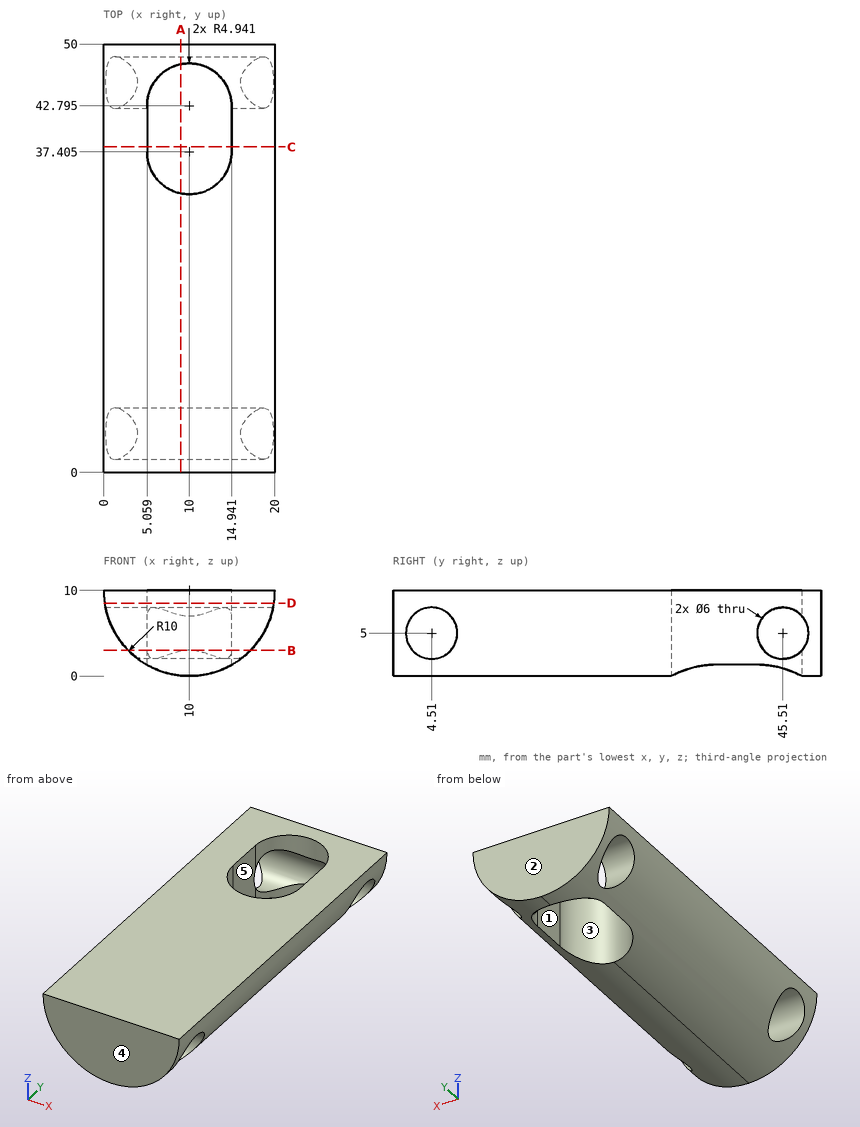
Verification items for this drawing (mm, ordinates from the low corner). A direction names the side the tool comes from. Coordinates: 2 decimals unless noted, no trailing zeros. Write each loop counter-clockwise with the first axis right and the second up, starting at its lowest first coordinate (ties: lowest second). Pieces come first, ordered by that corner, then holes. Notation, with made-up numbers: (1, 83) -> (43, 83) arc R27 cw to (43, 113) -> close; hole circle Ø3 at (4.25, 1.25). An arc over 180 degrees is marked (long way). Use CSV: the item, a comma, the result in double quotes. Start each with the question number.
Item 1: Thickness scan on line 1 (Y direction, x = 8.5, z = 5); line 2 (Y direction, x = 6.5, z = 5); line 3 (Y direction, x = 10.5, z = 1). Record the ranges inside material, lowest first.
Item 2: Depth check by flat-ended pin: pin 1 Ø4 at (y, z) = (24.5, 7) entering from -X; pin 2 Ø2 at (y, z) = (45, 2) entering from +X. Enter the tip coordinate at first touch or a pass-through.
Item 3: Cross-section at D-D, the plane z = 8.5. Record the cut outline in (x, y) (1 decimal).
Item 4: Set-up check for the marked faces 1 and 2: record each of +Z, -Z, +X, -X, +Y, -Y from which the full face is reachable in a straight line by a thin tool's end or side.
Item 5: Cross-section at B-B, the plane z = 3. Record the cut outline in (x, y) (1 decimal), plus the area to 3 significant figures.
Item 6: Cross-section at C-C, the plane y = 38. Record the cut outline in (x, z).
Item 7: Mould release check, pull along X, two halves, no side actions. Record for the marked faces 3, 4 and 5: released by +X, released by -X, zero draft, split by the parting line, or undercut.
Item 8: Cross-section at A-A, the plane x = 9. Record the cut outline in (y, z), plus the area to 3 significant figures.
Answers:
1,line 1,"0 to 1.51, 7.51 to 32.7, 48.51 to 50"
1,line 2,"0 to 1.51, 7.51 to 33.92, 48.51 to 50"
1,line 3,"0 to 32.49, 47.71 to 50"
2,pin 1,"x = 0.05"
2,pin 2,"x = 16.46"
3,outline,"(0.1, 0) -> (19.9, 0) -> (19.9, 50) -> (0.1, 50) -> close; hole (5.1, 37.4) arc R4.9 ccw to (14.9, 37.4) -> (14.9, 42.8) arc R4.9 ccw to (5.1, 42.8) -> close"
4,face 1,"+Z, -Z"
4,face 2,"+Z, -Z, +X, -X, +Y"
5,outline,"(2.9, 0) -> (17.1, 0) -> (17.1, 2.3) -> (2.9, 2.3) -> close; (2.9, 6.7) -> (17.1, 6.7) -> (17.1, 43.3) -> (14.9, 43.3) arc R4.9 cw to (14.9, 42.8) -> (14.9, 37.4) arc R4.9 cw to (5.1, 37.4) -> (5.1, 42.8) arc R4.9 cw to (5.1, 43.3) -> (2.9, 43.3) -> close; (2.9, 47.7) -> (17.1, 47.7) -> (17.1, 50) -> (2.9, 50) -> close"
5,area,"490 mm^2"
6,outline,"(0, 10) arc R10 ccw to (5.06, 1.31) -> (5.06, 10) -> close; (14.94, 1.31) arc R10 ccw to (20, 10) -> (14.94, 10) -> close"
7,face 3,"undercut"
7,face 4,"zero draft"
7,face 5,"undercut"
8,outline,"(0, 0.05) -> (32.57, 0.05) -> (32.57, 10) -> (0, 10) -> close; (47.63, 0.05) -> (50, 0.05) -> (50, 10) -> (47.63, 10) -> (47.63, 7.12) arc R3 cw to (47.63, 2.88) -> close; hole circle Ø6 at (4.51, 5)"
8,area,"317 mm^2"
